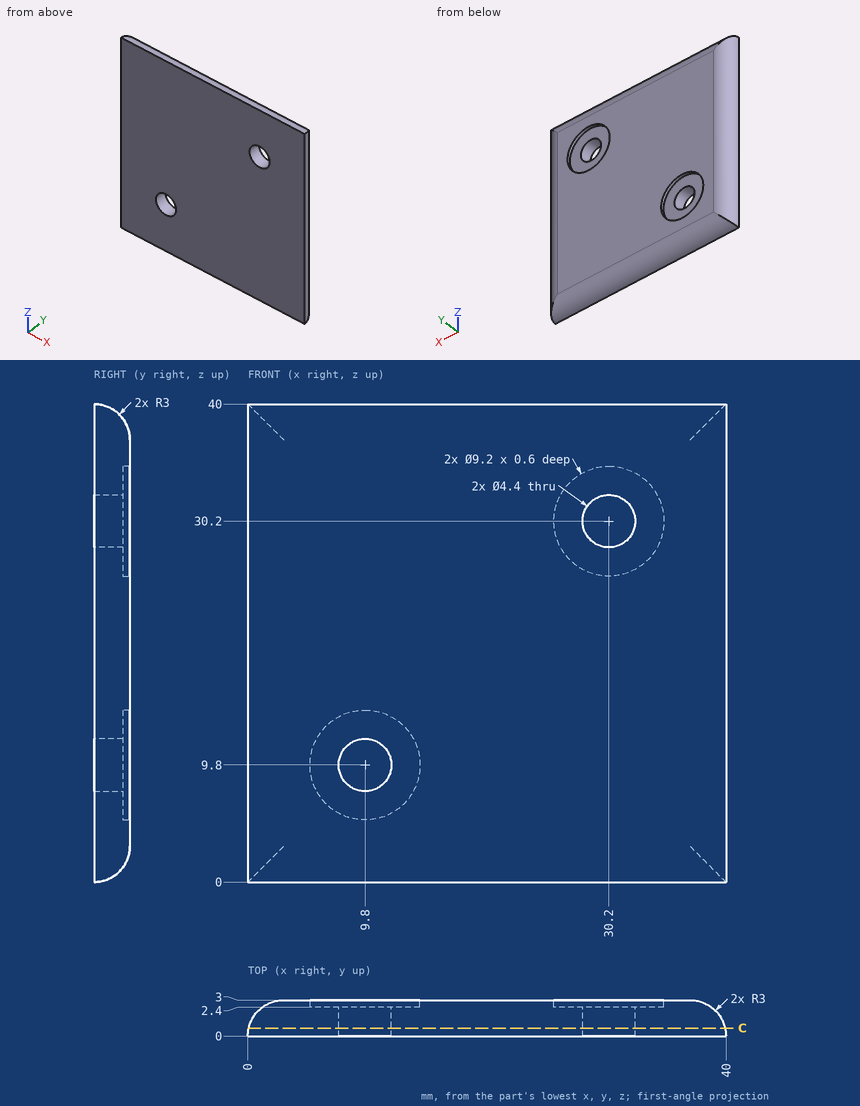
Job drawing, mm, ordinate dimensions from the low corner. One solid piece. Coordinates: 2 decimals unless noted, no trailing zeros. Loops run counter-clockwise (first coordinate to the right, second up) from the corner with the lowest first, then second, coordinate; pieces in that order, holes last. Notation, with made-up numbers: (54.25, -10) -> (75.25, -10) arc R33 ccw to (75.25, 27) -> close; hole circle Ø10 at (-5, 39.5). An arc over 180 degrees is marked (long way). One line per item, written item: value.
1. Flat gauge pins, fed straight in: P1, Ø8, axis at x = 15.5, z = 34, coming from the -Y side; P2, Ø7.5, axis at x = 9.8, z = 9.8, coming from the +Y side. Where does each tip first touch, or does it go through?
Answers:
P1: stops at y = 0
P2: stops at y = 2.4
2. Drill centre lines: line 1 (Y direction, x = 28.5, z = 32); line 2 (X direction, y = 2.65, z = 30.2); line 3 (Z direction, x = 8, y = 0.15) (1 decimal). Where is each one in solid material? Low to high. Write a range as [from, to].
Answers:
line 1: y = [0, 2.4]
line 2: x = [1.59, 25.6], [34.8, 38.41]
line 3: z = [0, 8.5], [11.1, 40]
3. Slice it at C-C on y = 0.65. Write the cut outline in (x, z), and give its area (3 significant figures).
Answers:
outline: (0.07, 0.07) -> (39.93, 0.07) -> (39.93, 39.93) -> (0.07, 39.93) -> close; hole circle Ø4.4 at (9.8, 9.8); hole circle Ø4.4 at (30.2, 30.2)
area: 1,560 mm^2
